Input: part model. Units: mm. Frame: model coordinates. Round coordinates to 2 decimals unless told otherwise and drop trailing zeros. Write each loop counter-clockwise with the first axis right and the second up, starting at its lowest first coordinate (ties: lowest second). Pieces come first, ordered by that corner, then holes. Notation, with made-up numbers: M -32,-15.5 L -11,-15.5 A18 cw -11,6.5 Z; hole C 39.25,76.25 d4. An arc over 180 degrees is marked long. Write each question's results on one line, items separated by ' | '. Start each with the question number.
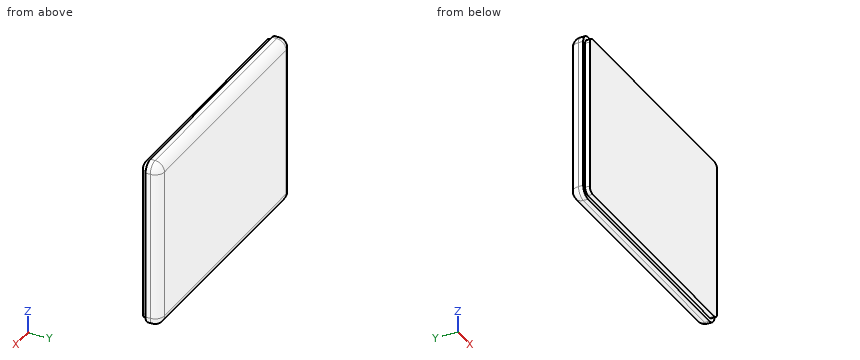
```python
from build123d import *

# Parameters (mm, degrees)
SKETCH1_W      = 270
SKETCH1_H      = 180
EXTRUDE1_DEPTH = 20
FILLET1_R      = 10
EXTRUDE3_DEPTH = 5


with BuildPart() as part:
    # Sketch1 → Extrude1 (new body)
    with BuildSketch(Plane(origin=(0, 0, 0), x_dir=(1, 0, 0), z_dir=(0, 1, 0))):
        Rectangle(SKETCH1_W, SKETCH1_H)
    extrude(amount=EXTRUDE1_DEPTH)

    # Fillet1
    fillet1_edges = [part.edges().sort_by_distance(p)[0] for p in [
        (-135, 20, 0),
        (0, 20, 90),
        (135, 20, 0),
        (0, 20, -90),
        (135, 10, 90),
        (-135, 10, 90),
        (-135, 10, -90),
        (135, 10, -90),
    ]]
    fillet(fillet1_edges, radius=FILLET1_R)

    # Sketch3 → Extrude3 (cut)
    with BuildSketch(Plane.XZ):
        with BuildLine():
            Line((125, 90), (-125, 90))
            ThreePointArc((-125, 90), (-132.071067812, 87.071067812), (-135, 80))
            Line((-135, 80), (-135, -80))
            ThreePointArc((-135, -80), (-132.071067812, -87.071067812), (-125, -90))
            Line((-125, -90), (125, -90))
            ThreePointArc((125, -90), (132.071067812, -87.071067812), (135, -80))
            Line((135, -80), (135, 80))
            ThreePointArc((135, 80), (132.071067812, 87.071067812), (125, 90))
        make_face()
        with BuildLine():
            Line((-131, 80), (-131, -80))
            ThreePointArc((-131, -80), (-129.242640687, -84.242640687), (-125, -86))
            Line((-125, -86), (125, -86))
            ThreePointArc((125, -86), (129.242640687, -84.242640687), (131, -80))
            Line((131, -80), (131, 80))
            ThreePointArc((131, 80), (129.242640687, 84.242640687), (125, 86))
            Line((125, 86), (-125, 86))
            ThreePointArc((-125, 86), (-129.242640687, 84.242640687), (-131, 80))
        make_face(mode=Mode.SUBTRACT)
    extrude(amount=-EXTRUDE3_DEPTH, mode=Mode.SUBTRACT)


solid = part.part
```
1. Cut plane B-B on z = 63. Output: boundary loops of the cut face in (x, y), and give its area (3 significant figures).
2. Cut plane A-A on x = 97.5. Output: boundary loops of the cut face in (y, z).
3. Line query: L1, parallel to X at y = 3.25, z = 67; L2, parallel to Z at x = 32, y = 11; L3, parallel to Z at x = 68, y = 4.5. Output: solid intervals per line, ascending. Write a range as from..to.
4. Contact query for flat-ended pins moving along their axis: P1, Ø2, axis at x = -8.5, y = 17, coming from the +Z side; P2, Ø6, axis at y = 17, z = -41.5, coming from the -X side; P3, Ø2.5, axis at x = -50.5, y = 3.5, coming from the +Z side. Output: stop coordinate, or through.
5. Cut plane C-C on y = 15. Output: boundary loops of the cut face in (x, z), and give its area (3 significant figures).
Answers follow:
1) outline: M -135,5 L -131,5 L -131,0 L 131,0 L 131,5 L 135,5 L 135,10 A10 ccw 125,20 L -125,20 A10 ccw -135,10 Z | area: 5,320 mm2
2) outline: M 0,-86 L 5,-86 L 5,-90 L 10,-90 A10 ccw 20,-80 L 20,80 A10 ccw 10,90 L 5,90 L 5,86 L 0,86 Z
3) L1: x = -131..131 | L2: z = -89.95..89.95 | L3: z = -86..86
4) P1: stops at z = 88 | P2: stops at x = -134.17 | P3: stops at z = 86
5) outline: M -133.66,-80 A8.66 ccw -125,-88.66 L 125,-88.66 A8.66 ccw 133.66,-80 L 133.66,80 A8.66 ccw 125,88.66 L -125,88.66 A8.66 ccw -133.66,80 Z | area: 47,300 mm2
